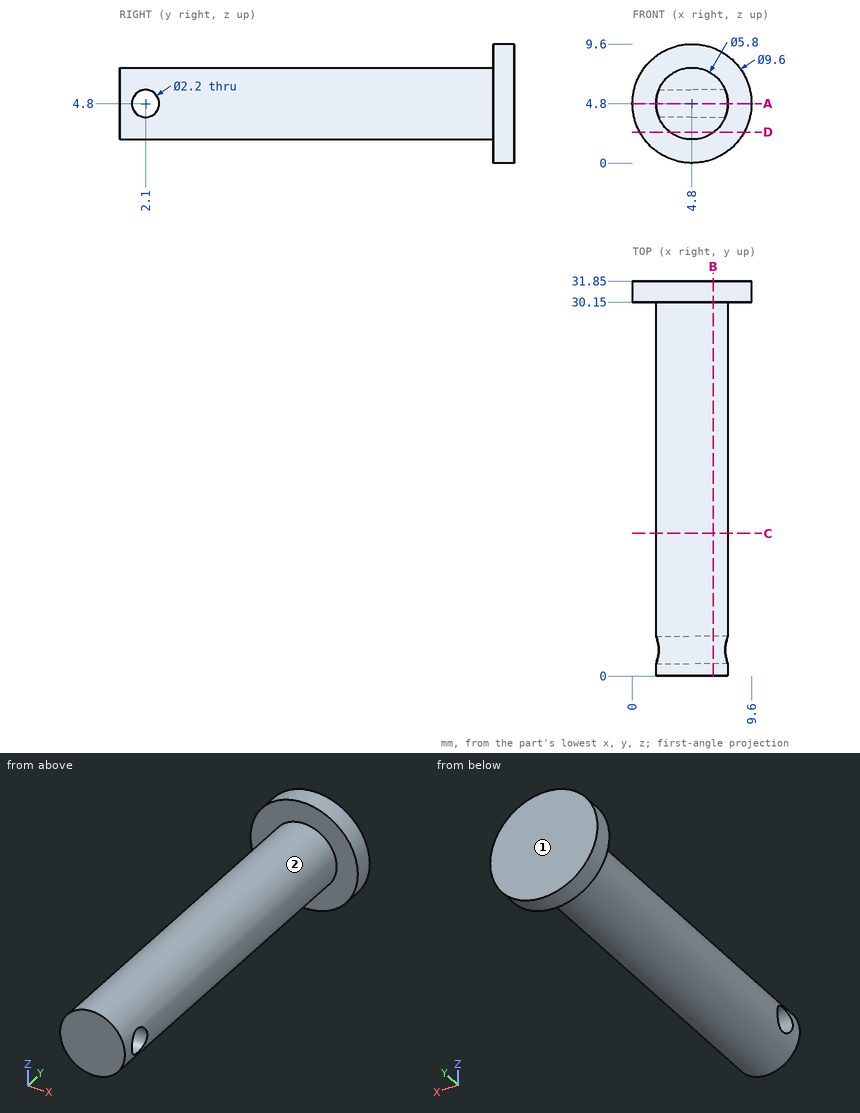
For this review, use the dimensioned drawing (mm, ordinates from the lowest corner) and the shaded views. A direction names the side the tool comes from. Coordinates: 2 decimals unless noted, no trailing zeros. Write each loop counter-clockwise with the first axis right and the second up, starting at its lowest first coordinate (ties: lowest second). Pieces come first, ordered by that corner, then holes. Notation, with made-up numbers: (69, 6) - (99, 6) arc R19 ccw to (99, 10) - close; hole circle Ø11 at (32.25, 14). An arc over 180 degrees is marked (long way). Answer as a JSON object with one key per item and string values. Group by question number.
1. Add section A-A (z = 4.8). Give the boundary of the cut face in (x, y), plus the area to 3 significant figures.
2. To check wall thickness, follow probe 1 along Y at (x, z) = (5.7, 4.8); probe 2 along Y at (x, z) = (0.75, 5.5); probe 3 along Z at (x, y) = (6, 2). State the ranges of each line that lie inside material, in increasing order.
3. Clearance check with flat-ended pins moving along their axes: pin 1 Ø3 at (x, y) = (2.5, 26.5) entering from -Z; pin 2 Ø5 at (y, z) = (3.5, 1.5) entering from +X; pin 3 Ø4 at (x, y) = (6, 14) entering from +Z. State where each tip first meets the part, or that it passes through.
4. Add section D-D (z = 2.5). Give the boundary of the cut face in (x, y), plus the area to 3 significant figures.
5. Add section C-C (y = 11.5). Give the boundary of the cut face in (x, z).
6. Add section B-B (x = 6.5). Give the boundary of the cut face in (y, z), plus the area to 3 significant figures.
7. Machinability: for the marked faces 1 and 2, which of the approach directions +Z, -Z, +X, -X, +Y, -Y give a long, thin tool a straight path to every point of the face, cutting with its end or side? Answer none if there is none.
Findings:
{
 "1": {"outline": "(0, 30.15) - (1.9, 30.15) - (1.9, 3.2) - (7.7, 3.2) - (7.7, 30.15) - (9.6, 30.15) - (9.6, 31.85) - (0, 31.85) - close; (1.9, 0) - (7.7, 0) - (7.7, 1) - (1.9, 1) - close", "area": "178 mm²"},
 "2": {"probe 1": "0 to 1, 3.2 to 31.85", "probe 2": "30.15 to 31.85", "probe 3": "2.16 to 3.7, 5.9 to 7.44"},
 "3": {"pin 1": "z = 2.01", "pin 2": "x = 7.59", "pin 3": "z = 7.7"},
 "4": {"outline": "(0.59, 30.15) - (3.03, 30.15) - (3.03, 0) - (6.57, 0) - (6.57, 30.15) - (9.01, 30.15) - (9.01, 31.85) - (0.59, 31.85) - close", "area": "121 mm²"},
 "5": {"outline": "circle Ø5.8 at (4.8, 4.8)"},
 "6": {"outline": "(0, 2.45) - (30.15, 2.45) - (30.15, 0.31) - (31.85, 0.31) - (31.85, 9.29) - (30.15, 9.29) - (30.15, 7.15) - (0, 7.15) - close; hole circle Ø2.2 at (2.1, 4.8)", "area": "153 mm²"},
 "7": {"face 1": "+Z, -Z, +X, -X, +Y", "face 2": "-Y"}
}
